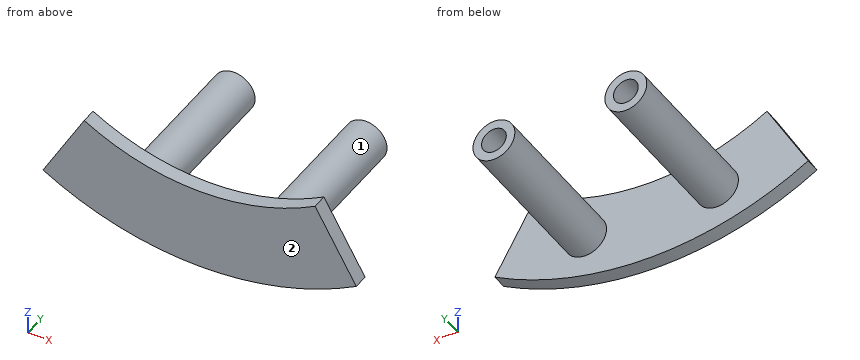
from build123d import *

# Parameters (mm, degrees)
BOSS_EXTRUDE1_DEPTH = 1.8
SKETCH2_R           = 2.54
BOSS_EXTRUDE2_DEPTH = 18.7
SKETCH5_R           = 1.5
CUT_EXTRUDE1_DEPTH  = 3


with BuildPart() as part:
    # Sketch1 → Boss-Extrude1 (new body)
    with BuildSketch(Plane(origin=(0, 0, 0), x_dir=(1, 0, 0), z_dir=(0, 1, 0))):
        with BuildLine():
            Line((-19, 32.908965344), (-14, 24.248711306))
            ThreePointArc((-14, 24.248711306), (0, 28), (14, 24.248711306))
            Line((14, 24.248711306), (19, 32.908965344))
            ThreePointArc((19, 32.908965344), (0, 38), (-19, 32.908965344))
        make_face()
    extrude(amount=BOSS_EXTRUDE1_DEPTH)

    # Sketch2 → Boss-Extrude2 (add)
    with BuildSketch(Plane(origin=(0, 1.8, 0), x_dir=(1, 0, 0), z_dir=(0, 1, 0))):
        with Locations(Location((-8, 32, 0), (0, 0, 90))):
            Circle(SKETCH2_R)
        with Locations(Location((8, 32, 0), (0, 0, 90))):
            Circle(SKETCH2_R)
    extrude(amount=BOSS_EXTRUDE2_DEPTH)

    # Sketch5 → Cut-Extrude1 (cut)
    with BuildSketch(Plane(origin=(0, 20.5, 0), x_dir=(1, 0, 0), z_dir=(0, 1, 0))):
        with Locations(Location((-8, 32, 0), (0, 0, 270))):
            Circle(SKETCH5_R)
        with Locations(Location((8, 32, 0), (0, 0, 270))):
            Circle(SKETCH5_R)
    extrude(amount=-CUT_EXTRUDE1_DEPTH, mode=Mode.SUBTRACT)


solid = part.part
Source: CAD feature listing. Evaluate the final solid. Frame: model axes, mm. Face numbers are marked on the shaded views. Give positions to 0.01 mm unless a question says otherwise; leave off trailing zeros. Write each loop counter-clockwise with the first axis right and the second up, starting at its lowest first coordinate (ties: lowest second). Pieces come first, ordered by that corner, then holes. Notation, with made-up numbers: (24.5, 76.25) -> (74.5, 76.25) arc R13 cw to (74.5, 97.25) -> close; hole circle Ø6 at (34.25, 66). An arc over 180 degrees is marked (long way). Return JSON: item names as keys, results as strings. Group by question number.
1. Material intervals for line 1 (X direction, y = 19.5, z = -32); line 2 (Y direction, x = 6.5, z = -27.5); line 3 (X direction, y = 18.75, z = -33), sorted ascending. Write a range as from..to.
2. Section B-B, the plane x = 7. Output: boundary loops of the cut face in (y, z), then the cut area to 3 significant figures.
3. Section C-C, the plane y = 5.25. Output: boundary loops of the cut face in (x, z), then the cut area to 3 significant figures.
4. Section A-A, the plane z = -25.75. Output: boundary loops of the cut face in (x, y), then the cut area to 3 significant figures.
5. Section D-D, the plane z = -31.75. Output: boundary loops of the cut face in (x, y), then the cut area to 3 significant figures.
6. Pin query (flat end, axial travel): pin 1 Ø1.8 at (x, z) = (8, -32) entering from +Y; pin 2 Ø8 at (x, y) = (-0.5, 3.5) entering from +Z; pin 3 Ø6 at (y, z) = (9, -28.5) entering from +X. Return the tip coordinate at first contact, or that it passes through.
7. Mould query, pull axis X, two halves, no side actions, for the marked faces 1 and 2. Classes: +X half, -X half, draft (parallel to the pull), parting line (faces both ways), or undercut.
Determined:
{
 "1": {"line 1": "x = -10.54..-9.5, -6.5..-5.46, 5.46..6.5, 9.5..10.54", "line 2": "y = 0..1.8", "line 3": "x = -10.33..-9.12, -6.88..-5.67, 5.67..6.88, 9.12..10.33"},
 "2": {"outline": "(0, -37.35) -> (1.8, -37.35) -> (1.8, -34.33) -> (20.5, -34.33) -> (20.5, -33.12) -> (17.5, -33.12) -> (17.5, -30.88) -> (20.5, -30.88) -> (20.5, -29.67) -> (1.8, -29.67) -> (1.8, -27.11) -> (0, -27.11) -> close", "area": "99.0 mm2"},
 "3": {"outline": "circle Ø5.08 at (-8, -32); circle Ø5.08 at (8, -32)", "area": "40.5 mm2"},
 "4": {"outline": "(-14.87, 0) -> (-11, 0) -> (-11, 1.8) -> (-14.87, 1.8) -> close; (11, 0) -> (14.87, 0) -> (14.87, 1.8) -> (11, 1.8) -> close", "area": "13.9 mm2"},
 "5": {"outline": "(-18.33, 0) -> (18.33, 0) -> (18.33, 1.8) -> (10.53, 1.8) -> (10.53, 20.5) -> (9.48, 20.5) -> (9.48, 17.5) -> (6.52, 17.5) -> (6.52, 20.5) -> (5.47, 20.5) -> (5.47, 1.8) -> (-5.47, 1.8) -> (-5.47, 20.5) -> (-6.52, 20.5) -> (-6.52, 17.5) -> (-9.48, 17.5) -> (-9.48, 20.5) -> (-10.53, 20.5) -> (-10.53, 1.8) -> (-18.33, 1.8) -> close", "area": "237 mm2"},
 "6": {"pin 1": "stops at y = 17.5", "pin 2": "stops at z = -27.7", "pin 3": "stops at x = 10.49"},
 "7": {"face 1": "undercut", "face 2": "draft"}
}
